Can you work these out from the model? Positions are in its coordinate system, mm. Round coordinates to 2 decimals unless told otherwise and drop trailing zeros. Loops run counter-clockwise (first coordinate to the right, second up) from the corner with the lowest first, then second, coordinate; pieces in that order, holes last.
(1) I want a section at A-A on z = 9. Write out the boundary of the cut face in (x, y), plus the area to 3 significant figures.
(2) Will this pin go through, and if not, where does the flat tip stop? pin 1 Ø8 at (y, z) = (-16.5, 10.5) entering from +X (3 decimals).
(3) If I drill on line 1 along Y through (x, z) = (23, 17); line 2 along Y through (x, z) = (24.3, 18); line 3 along Z through (x, y) = (22.05, -6), over which ranges is the centre line in solid material (lowest first)?
(4) I want a section at B-B on y = 2.5. Write out the boundary of the cut face in (x, z), plus the area to 3 significant figures.
Autodesk Inventor part; units mm, degrees
ref_plane "作業平面1" through (-53.6786, -65.4442, 30.5) normal (0, 0, -1) x (0.7071068, 0.7071068, 0)
ref_plane "YZ Plane" through (0, 0, 0) normal (1, 0, 0) x (0, 1, 0)
ref_plane "XZ Plane" through (0, 0, 0) normal (0, 1, 0) x (-1, 0, 0)
sketch "スケッチ1" plane through (0, 0, 0) normal (0, 0, 1) x (1, 0, 0)
  circle A0 centre (23.0793, 24.731) radius 1.1
  circle A1 centre (23.0793, -24.731) radius 1.1
  line L0 (24.5793, 27.731) -> (21.5793, 27.731)
  line L1 (21.5793, 27.731) -> (21.5793, -27.731)
  line L2 (21.5793, -27.731) -> (24.5793, -27.731)
  line L3 (24.5793, -27.731) -> (24.5793, 27.731)
  point P0 (0, 0)
  point P1 (23.0793, 27.731)
  dimension "d0" = 3
  dimension "d1" = 3
  dimension "d2" = 3
ref_plane "作業平面1" through (-53.6786, -65.4442, 30.5) normal (0, 0, -1) x (0.7071068, 0.7071068, 0)
extrude "押し出し1" add sketch "スケッチ1" along normal up to surface (30.5 mm away) contours A0 | A1 | L3 L2 L1 L0
sketch "スケッチ2" plane through (0, 0, 0) normal (0, 0, -1) x (-1, 0, 0)
  circle A0 centre (-23.0793, 24.731) radius 1.1
  circle A1 centre (-23.0793, -24.731) radius 1.1
  point P0 (0, 0)
hole "穴1" at (23.0793, 24.731, 0) at (23.0793, -24.731, 0) direction (0, 0, 1) diameter 1.567 end through all
sketch "スケッチ3" plane through (24.5793, -27.731, 0) normal (1, 0, 0) x (0, 0, -1)
  line L0 (-30.5, 0) -> (-30.5, 55.4619)
  line L1 (0, 0) -> (-30.5, 0)
  line L2 (0, 0) -> (0, 55.4619)
  line L3 (0, 55.4619) -> (-30.5, 55.4619)
  line L4 (-4, 51.4619) -> (-4, 4)
  line L5 (-4, 4) -> (-26.5, 4)
  line L6 (-26.5, 4) -> (-26.5, 51.4619)
  line L7 (-26.5, 51.4619) -> (-4, 51.4619)
  point P0 (0, 27.731)
  dimension "d12" = 4
extrude "押し出し2" cut sketch "スケッチ3" against normal through all contours L4 L5 L6 L7
fillet "フィレット1" radius 2 4 edges at (23.0793, 23.731, 26.5) (23.0793, 23.731, 4) (23.0793, -23.731, 26.5) (23.0793, -23.731, 4)
sketch "スケッチ4" plane through (24.5793, -27.731, 0) normal (1, 0, 0) x (0, 0, -1)
  line L0 (0, 53.2454) -> (0, 51.6784) construction
  line L1 (0, 3.7835) -> (0, 2.2165) construction
  line L2 (-30.5, 4.1) -> (-30.5, 1.9) construction
  line L3 (-30.5, 51.6784) -> (-30.5, 53.2454) construction
  circle A0 centre (-31.5, 52.4619) radius 1.1
  line L4 (0, 27.731) -> (-30.5, 27.731) construction
  line L5 (-30.5, 0) -> (-30.5, 55.4619) construction
  line L6 (-15.25, 27.731) -> (-15.25, 0) construction
  line L7 (0, 0) -> (-30.5, 0) construction
  circle A1 centre (-31.5, 3) radius 1.1
  circle A2 centre (1, 52.4619) radius 1.1
  circle A3 centre (1, 3) radius 1.1
  point P0 (-30.5, 52.4619)
  dimension "d16" = 2.2
  dimension "d17" = 1
extrude "押し出し3" cut sketch "スケッチ4" against normal through all
equation "\"d2\" = d1"
properties part number "kosinosita"
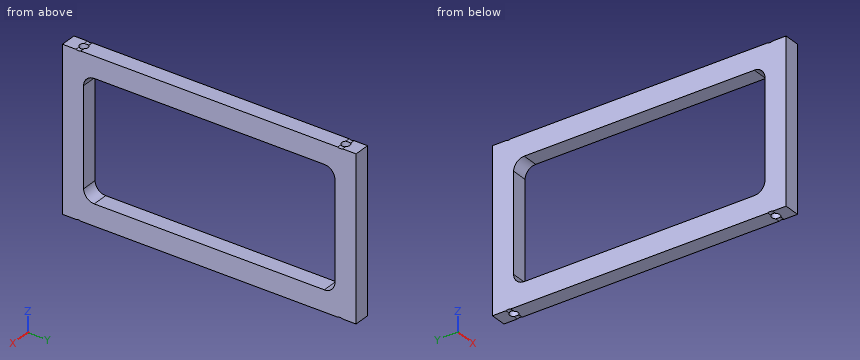
Filled sheet:
1. outline: (21.58, -27.73) - (24.58, -27.73) - (24.58, -23.73) - (21.58, -23.73) - close; (21.58, 23.73) - (24.58, 23.73) - (24.58, 27.73) - (21.58, 27.73) - close; hole circle Ø1.57 at (23.08, -24.73); hole circle Ø1.57 at (23.08, 24.73)
1. area: 20.1 mm2
2. pin 1: passes through
3. line 1: y = -27.73 to -25.51, -23.95 to -23.73, 23.73 to 23.95, 25.51 to 27.73
3. line 2: y = -27.73 to -23.73, 23.73 to 27.73
3. line 3: z = 0 to 4, 26.5 to 30.5
4. outline: (21.58, 0) - (24.58, 0) - (24.58, 4) - (21.58, 4) - close; (21.58, 26.5) - (24.58, 26.5) - (24.58, 30.5) - (21.58, 30.5) - close
4. area: 24.0 mm2
